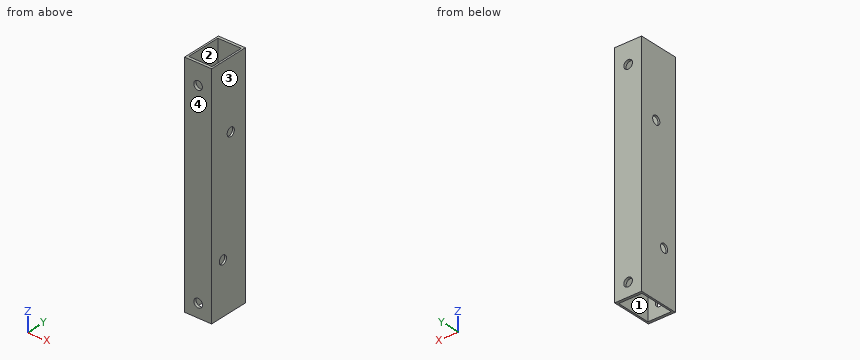
```python
from build123d import *

# Parameters (mm, degrees)
SKETCH_1_W          = 10
SKETCH_1_H          = 15
SKETCH_1_W_2        = 8.666666666
SKETCH_1_H_2        = 13
EXTRUDE_1_DEPTH     = 85
SKETCH_3_R          = 1.6
CUT_EXTRUDE_2_DEPTH = 87.458082329
SKETCH_4_R          = 1.6
CUT_EXTRUDE_3_DEPTH = 86.914201387


with BuildPart() as part:
    # ｽｹｯﾁ1 → ﾎﾞｽ - 押し出し1 (new body)
    with BuildSketch(Plane.XY):
        Rectangle(SKETCH_1_W, SKETCH_1_H)
        Rectangle(SKETCH_1_W_2, SKETCH_1_H_2, mode=Mode.SUBTRACT)
    extrude(amount=EXTRUDE_1_DEPTH)

    # ｽｹｯﾁ3 → ｶｯﾄ - 押し出し2 (cut, through all)
    with BuildSketch(Plane(origin=(0, 7.5, 0), x_dir=(1, 0, 0), z_dir=(0, 1, 0))):
        with Locations(Location((0, -77.5, 0), (0, 0, 270))):
            Circle(SKETCH_3_R)
        with Locations(Location((0, -5, 0), (0, 0, 270))):
            Circle(SKETCH_3_R)
    extrude(amount=-CUT_EXTRUDE_2_DEPTH, mode=Mode.SUBTRACT)

    # ｽｹｯﾁ4 → ｶｯﾄ - 押し出し3 (cut, through all)
    with BuildSketch(Plane.ZY.offset(5)):
        with Locations((60, 1)):
            Circle(SKETCH_4_R)
        with Locations((19, -2.5)):
            Circle(SKETCH_4_R)
    extrude(amount=-CUT_EXTRUDE_3_DEPTH, mode=Mode.SUBTRACT)


solid = part.part
```
Geometry: final body of the model. Coordinates: model frame, mm. Face numbers are marked on the shaded views. Give positions to 0.01 mm unless a question says otherwise; leave off trailing zeros. Loops run counter-clockwise (first coordinate to the right, second up) from the corner with the lowest first, then second, coordinate; pieces in that order, holes last. Notation, with made-up numbers: (89.25, 36) -> (134.25, 36) arc R18 ccw to (134.25, 59) -> close; hole circle Ø11 at (89.25, 68). An arc over 180 degrees is marked (long way). Return JSON: item names as keys, results as strings.
Item 1: Mould query, pull axis X, two halves, no side actions, for the marked faces 1, 2, 3 and 4. Classes: released by +X, released by -X, zero draft, split by the parting line, or undercut.
Filled in:
{"face 1": "undercut", "face 2": "undercut", "face 3": "released by +X", "face 4": "zero draft"}
Item 2: Section C-C, the plane z = 60. Output: boundary loops of the cut face in (x, y), plus the area to 3 significant figures.
Filled in:
{"outline": "(-5, -7.5) -> (5, -7.5) -> (5, -0.6) -> (4.33, -0.6) -> (4.33, -6.5) -> (-4.33, -6.5) -> (-4.33, -0.6) -> (-5, -0.6) -> close; (-5, 2.6) -> (-4.33, 2.6) -> (-4.33, 6.5) -> (4.33, 6.5) -> (4.33, 2.6) -> (5, 2.6) -> (5, 7.5) -> (-5, 7.5) -> close", "area": "33.1 mm^2"}
Item 3: Section D-D, the plane y = 4. Output: boundary loops of the cut face in (x, z), plus the area to 3 significant figures.
Filled in:
{"outline": "(-5, 0) -> (-4.33, 0) -> (-4.33, 85) -> (-5, 85) -> close; (4.33, 0) -> (5, 0) -> (5, 85) -> (4.33, 85) -> close", "area": "113 mm^2"}
Item 4: Section B-B, the plane x = 3.5. Output: boundary loops of the cut face in (y, z), plus the area to 3 significant figures.
Filled in:
{"outline": "(-7.5, 0) -> (-6.5, 0) -> (-6.5, 85) -> (-7.5, 85) -> close; (6.5, 0) -> (7.5, 0) -> (7.5, 85) -> (6.5, 85) -> close", "area": "170 mm^2"}
Item 5: Line query: line 1 (Y direction, x = 1.25, z = 35.5); line 2 (Y direction, x = 4.65, z = 19); line 3 (X direction, y = -7.15, z = 5). Output: solid intervals per line, ascending.
Filled in:
{"line 1": "-7.5 to -6.5, 6.5 to 7.5", "line 2": "-7.5 to -4.1, -0.9 to 7.5", "line 3": "-5 to -1.6, 1.6 to 5"}
Item 6: Section A-A, the plane y = -2.5. Output: boundary loops of the cut face in (x, z), plus the area to 3 significant figures.
Filled in:
{"outline": "(-5, 0) -> (-4.33, 0) -> (-4.33, 17.4) -> (-5, 17.4) -> close; (-5, 20.6) -> (-4.33, 20.6) -> (-4.33, 85) -> (-5, 85) -> close; (4.33, 0) -> (5, 0) -> (5, 17.4) -> (4.33, 17.4) -> close; (4.33, 20.6) -> (5, 20.6) -> (5, 85) -> (4.33, 85) -> close", "area": "109 mm^2"}
Item 7: Pin query (flat end, axial travel): P1, Ø2.5, axis at x = 0, z = 77.5, coming from the -Y side. Return the tip coordinate at first contact, or that it passes through.
Filled in:
{"P1": "through"}
